Geometry check sheet. Reference: drawing and pictorial views, mm from the part's lowest x, y, z. A direction names the side the tool comes from. Round coordinates to 2 decimals unless told otherwise and drop trailing zeros. Order: outer loops, then holes, each group sorted by start corner. A loop starts at its lowest first (then second) coordinate and runs counter-clockwise, first axis right, second up. Notation, with made-up numbers: (-3.75, 25) -> (9.25, 25) arc R17 ccw to (9.25, 50) -> close; hole circle Ø7 at (-35.75, 63). An arc over 180 degrees is marked (long way). Return JSON: item names as keys, results as strings. Group by question number.
1) Section check A-A on z = 19. Enter the section's corners in (x, y), plus the area to 3 significant figures.
2) Tool access check on the marked faces 1 and 2. Record the directions out of +Z, -Z, +X, -X, +Y, -Y that give a thin tool (end or side, any length) a straight path to the whole face; none if there is none.
3) Draft check along X on the marked faces 3, 4, 5 and 6. Enter one of: pulls with the +X half, pulls with the -X half, needs draft (parallel to the pull), parting line crosses it, or undercut.
4) Section check D-D on y = 85. State how many separate pieces and enclosed holes the cut face has, plus the area to 3 significant figures.
5) Section check C-C on x = 88.9. Enter the section's corners in (y, z) (1 decimal).
6) Depth check by flat-ended pin: pin 1 (8 mm diameter, centred on x = 69.5, y = 140, fed in from +Z) (3 decimals); pin 2 (10 mm diameter, centred on x = 22.5, z = 54.5, fed in from +Y); pin 3 (4 mm diameter, centred on x = 33, z = 26.5, fed in from -Y). Enter the tip coordinate at first touch or a pass-through.
7) Scan lines: L1, parallel to Y at x = 88, z = 2 (1 decimal); L2, parallel to X at y = 80.5, z = 57; L3, parallel to Z at x = 118.5, y = 98 (1 decimal). Record each from-to range of solid material in increasing order.
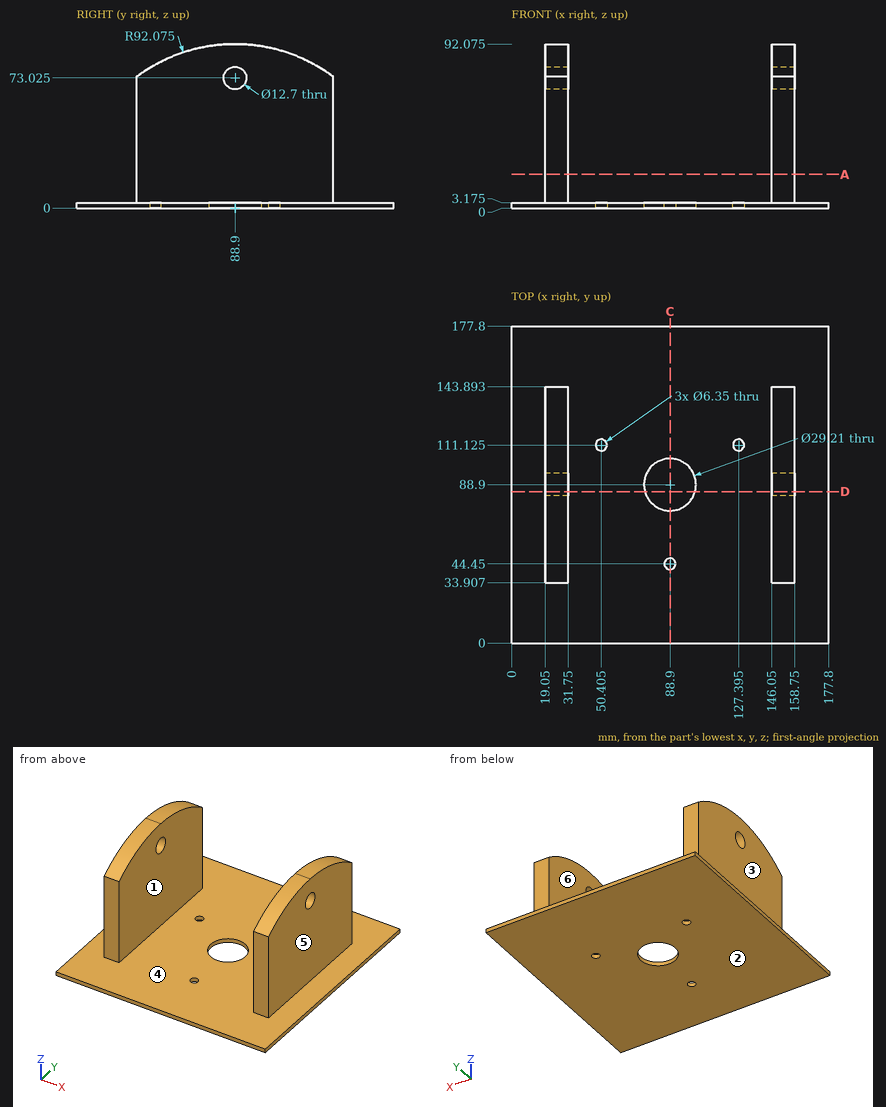
Check result:
{
 "1": {"outline": "(19.05, 33.91) -> (31.75, 33.91) -> (31.75, 143.89) -> (19.05, 143.89) -> close; (146.05, 33.91) -> (158.75, 33.91) -> (158.75, 143.89) -> (146.05, 143.89) -> close", "area": "2,790 mm^2"},
 "2": {"face 1": "+Z, +Y, -Y", "face 2": "-Z, +X, -X, +Y, -Y"},
 "3": {"face 3": "pulls with the -X half", "face 4": "undercut", "face 5": "pulls with the +X half", "face 6": "undercut"},
 "4": {"separate pieces": "4", "enclosed holes": "0", "area": "2,480 mm^2"},
 "5": {"outline": "(0, 0) -> (41.3, 0) -> (41.3, 3.2) -> (0, 3.2) -> close; (47.6, 0) -> (74.3, 0) -> (74.3, 3.2) -> (47.6, 3.2) -> close; (103.5, 0) -> (177.8, 0) -> (177.8, 3.2) -> (103.5, 3.2) -> close"},
 "6": {"pin 1": "z = 3.175", "pin 2": "y = 143.89", "pin 3": "y = 33.91"},
 "7": {"L1": "0 to 41.4, 47.5 to 74.3, 103.5 to 177.8", "L2": "19.05 to 31.75, 146.05 to 158.75", "L3": "0 to 3.2"}
}
